Design review of the part built by this model. Coordinates are the model's own, in mm. A direction names the side the tool comes from. Give positions to 0.01 mm unless a question says otherwise; leave off trailing zeros. Write each loop counter-clockwise with the first axis right and the second up, starting at its lowest first coordinate (ties: lowest second). Pieces come first, ordered by that corner, then holes. Notation, with made-up numbers: (39.5, 89.25) - (63.5, 89.25) arc R24 cw to (63.5, 113.25) - close; hole circle Ø8 at (65.25, 69.25). An arc over 180 degrees is marked (long way). Use a Markdown table: item, result. Add a question column.
```python
from build123d import *

# Parameters (mm, degrees)
BOSS_EXTRUDE1_START            = 2
BOSS_EXTRUDE1_DEPTH            = 10
CBORE_FOR_M3_SHCS2_D           = 3.4
CBORE_FOR_M3_SHCS2_CBORE_D     = 6.5
CBORE_FOR_M3_SHCS2_CBORE_DEPTH = 3
FILLET1_R                      = 1


with BuildPart() as part:
    # Sketch1 → Boss-Extrude1 (new body)
    with BuildSketch(Plane.XY.offset(BOSS_EXTRUDE1_START)):
        with BuildLine():
            Line((-12, 6), (12, 6))
            ThreePointArc((12, 6), (18, 0), (12, -6))
            Line((12, -6), (-12, -6))
            ThreePointArc((-12, -6), (-18, 0), (-12, 6))
        make_face()
    extrude(amount=BOSS_EXTRUDE1_DEPTH)

    # CBORE for M3 SHCS2 (through all)
    with Locations(Plane.XY.offset(12)):
        with Locations((-12, 0), (12, 0)):
            CounterBoreHole(CBORE_FOR_M3_SHCS2_D / 2, CBORE_FOR_M3_SHCS2_CBORE_D / 2, CBORE_FOR_M3_SHCS2_CBORE_DEPTH)

    # Fillet1
    fillet1_edges = [part.edges().sort_by_distance(p)[0] for p in [
        (18, 0, 12),
        (0, 6, 12),
        (8.75, 0, 12),
        (-15.25, 0, 12),
        (-18, 0, 12),
        (0, 6, 2),
        (18, 0, 2),
        (0, -6, 2),
        (-18, 0, 2),
        (0, -6, 12),
    ]]
    fillet(fillet1_edges, radius=FILLET1_R)

    # Sketch13 → Cut-Revolve1 (revolve, cut)
    with BuildSketch(Plane(origin=(0, 0, 0), x_dir=(0, 0, -1), z_dir=(1, 0, 0))):
        Polygon((0, 6), (0, -6), (8, -6), (8, -3), (6, -3), (6, 3), (8, 3), (8, 6), align=None)
    revolve(axis=Axis((0, 6, 0), (0, -1, 0)), mode=Mode.SUBTRACT)


solid = part.part
```
(1) Insertion check: pin 1 (7 mm diameter, centred on x = 13.5, y = 0, fed in from +Z); pin 2 (2 mm diameter, centred on y = 3, z = 11, fed in from -X); pin 3 (3 mm diameter, centred on x = -1.5, z = 5, fed in from -Y); pin 4 (4 mm diameter, centred on x = 12, y = 0, fed in from +Z). Each pin has a flat end and moves straight along its axis. Give the tip position at first contact, or say it passes through.
(2) Mouldability with a two-part tool opening along Y and no side actions: class faces 6 (the face through (0, 6, 9)), 7 (the face through (13.4, -1.4, 9)), 8 (the face through (0, -6, 9)), 9 (the face through (10.38, 0.51, 5.45)) as +Y half, -Y half, draft (parallel to the pull), parting line (faces both ways), or undercut.
(3) For line 1 along Y through (x, z) = (-12, 4); line 2 along X through (y, z) = (-0.25, 11.5); line 3 along Y through (x, z) = (12, 10.15), list the stretches that pass through material, from the lowest coordinate up.
(4) Add section B-B (z = 5.5). State the section outline as (x, y) points.
(5) Tool access review of faces 1 (the face through (0.1, -3, 6.4)), 2 (the face through (-9.676, 5.715, 2.301)), 3 (the face through (-0.168, -5.715, 11.699)), 4 (the face through (0.1, 3, 6.3)), 5 (the face through (-15.247, 0.143, 10.014)): name each direction out of +Z, -Z, +X, -X, +Y, -Y from which nothing blocks a thin tool from reaching the whole face with its end or side.
(6) Add section C-C (x = 3). State the section outline as (y, z) points.
(7) Add section A-A (y = 0). Count the separate pieces of the cut face and the enclosed holes in it, and give its area (3 significant figures).
Answers follow:
| question | item | result |
|---|---|---|
| 1 | pin 1 | z = 12 |
| 1 | pin 2 | x = -17.66 |
| 1 | pin 3 | y = -3 |
| 1 | pin 4 | z = 9 |
| 2 | face 6 | +Y half |
| 2 | face 7 | undercut |
| 2 | face 8 | -Y half |
| 2 | face 9 | undercut |
| 3 | line 1 | -6 to -1.7, 1.7 to 6 |
| 3 | line 2 | -17.86 to -15.37, -8.63 to 8.63, 15.37 to 17.86 |
| 3 | line 3 | -6 to -3.25, 3.25 to 6 |
| 4 | outline | (-12, -6) - (-5.81, -6) - (-5.81, -3) - (-2.4, -3) - (-2.4, 3) - (-5.81, 3) - (-5.81, 6) - (-12, 6) arc R6 ccw to start; (2.4, -3) - (5.81, -3) - (5.81, -6) - (12, -6) arc R6 ccw to (12, 6) - (5.81, 6) - (5.81, 3) - (2.4, 3) - close; hole circle Ø3.4 at (-12, 0); hole circle Ø3.4 at (12, 0) |
| 5 | face 1 | -Z, -Y |
| 5 | face 2 | -Z, +X, -X, +Y |
| 5 | face 3 | +Z, +X, -X, -Y |
| 5 | face 4 | -Z, +Y |
| 5 | face 5 | +Z |
| 6 | outline | (-6, 7.42) - (-3, 7.42) - (-3, 5.2) - (3, 5.2) - (3, 7.42) - (6, 7.42) - (6, 11) arc R1 ccw to (5, 12) - (-5, 12) arc R1 ccw to (-6, 11) - close |
| 7 | separate pieces | 3 |
| 7 | enclosed holes | 0 |
| 7 | area | 239 mm^2 |
